```python
from build123d import *

# Parameters (mm, degrees)
SKETCH1_R           = 38.1
BOSS_EXTRUDE1_DEPTH = 152.4
BOSS_EXTRUDE1_TAPER = 2
FILLET1_R           = 12.7
SKETCH2_R           = 50.8
BOSS_EXTRUDE2_DEPTH = 12.7
FILLET2_R           = 6.35


with BuildPart() as part:
    # Sketch1 → Boss-Extrude1 (new body)
    with BuildSketch(Plane(origin=(0, 0, 0), x_dir=(1, 0, 0), z_dir=(0, 1, 0))):
        Circle(SKETCH1_R)
    extrude(amount=BOSS_EXTRUDE1_DEPTH, taper=BOSS_EXTRUDE1_TAPER)

    # Fillet1
    fillet1_edges = [part.edges().sort_by_distance(p)[0] for p in [
        (-32.778074729, 152.4, 0),
    ]]
    fillet(fillet1_edges, radius=FILLET1_R)

    # Sketch2 → Boss-Extrude2 (add)
    with BuildSketch(Plane(origin=(0, 0, 0), x_dir=(1, 0, 0), z_dir=(0, 1, 0))):
        Circle(SKETCH2_R)
    extrude(amount=BOSS_EXTRUDE2_DEPTH)

    # Fillet2
    fillet2_edges = [part.edges().sort_by_distance(p)[0] for p in [
        (-50.8, 12.7, 0),
    ]]
    fillet(fillet2_edges, radius=FILLET2_R)


solid = part.part
```
Verification items for the finished model (mm, model axes). A direction names the side the tool comes from. Coordinates: 2 decimals unless noted, no trailing zeros. Order: outer loops, then holes, each group sorted by start corner. A loop starts at its lowest first (then second) coordinate and runs counter-clockwise, first axis right, second up. Notation, with made-up numbers: (64.5, 86) -> (109.5, 86) arc R28 cw to (109.5, 125) -> close; hole circle Ø4 at (15, -26). An arc over 180 degrees is marked (long way). Put each result on its own line as item: value. Start each with the question number.
1) Tool access check on faces 1 (the flat face through (-1, 0, -1)), 2 (the flat face through (-33, 12.7, -20)). Record the directions out of +Z, -Z, +X, -X, +Y, -Y that give a thin tool (end or side, any length) a straight path to the whole face; none if there is none.
2) Cross-section at A-A (x = 0). Enter the section's corners in (y, z), plus the area to 3 significant figures.
3) Material ranges on L1, parallel to Y at x = -33, z = 21; L2, parallel to X at y = 45, z = -10; L3, parallel to Y at x = 12, z = 23, recorded low to high.
4) Cross-section at C-C (y = 124). Enter the section's corners in (x, z).
5) Go/stop test with flat-tipped pins: pin 1 (8 mm diameter, centred on y = 61, z = 35.5, fed in from -X); pin 2 (5 mm diameter, centred on y = 81.5, z = -12, fed in from -X); pin 3 (10 mm diameter, centred on y = 34, z = -7, fed in from -X); pin 4 (2 mm diameter, centred on x = 31, z = 2.5, fed in from -Y). Record where each tip stops, or that it passes through.
6) Cross-section at B-B (y = 44). Enter the section's corners in (x, z), plus the area to 3 significant figures.
Geometry check:
1. face 1: +Z, -Z, +X, -X, -Y
1. face 2: +Y
2. outline: (0, -50.8) -> (6.35, -50.8) arc R6.35 ccw to (12.7, -44.45) -> (12.7, -37.66) -> (140.14, -33.21) arc R12.7 ccw to (152.4, -20.51) -> (152.4, 20.51) arc R12.7 ccw to (140.14, 33.21) -> (12.7, 37.66) -> (12.7, 44.45) arc R6.35 ccw to (6.35, 50.8) -> (0, 50.8) -> close
2. area: 11,000 mm^2
3. L1: y = 0 to 12.7
3. L2: x = -35.13 to 35.13
3. L3: y = 0 to 151.18
4. outline: circle Ø67.54 at (0, 0)
5. pin 1: stops at x = -17.37
5. pin 2: stops at x = -33.96
5. pin 3: stops at x = -36.9
5. pin 4: stops at y = 0
6. outline: circle Ø73.13 at (0, 0)
6. area: 4,200 mm^2
